```python
from build123d import *

# Parameters (mm, degrees)
F1_DEPTH = 20
F3_D     = 4.55
F4_R     = 5


with BuildPart() as f1:
    # F0 (on Right) → F1 (new body)
    with BuildSketch(Plane.YZ):
        Polygon((-15.453118, 0), (0, 0), (0, 13.234019), (-7.305924, 13.234019), (-7.305924, 2.900996), (-15.453118, 2.900996), align=None)
        Polygon((0, 13.234019), (0, 0), (15.453118, 0), (15.453118, 2.900996), (7.305924, 2.900996), (7.305924, 13.234019), align=None)
    extrude(amount=F1_DEPTH)

    # F3 (through all)
    with Locations(Plane.YZ.offset(20)):
        with Locations((0, 7.294424)):
            Hole(F3_D / 2)

    # F4
    f4_edges = [f1.edges().sort_by_distance(p)[0] for p in [
        (10, 7.305924, 13.234019),
        (10, -7.305924, 13.234019),
    ]]
    fillet(f4_edges, radius=F4_R)


solid = f1.part
```
Design review of the part built by this model. Coordinates are the model's own, in mm. A direction names the side the tool comes from. Coordinates: 2 decimals unless noted, no trailing zeros. Order: outer loops, then holes, each group sorted by start corner. A loop starts at its lowest first (then second) coordinate and runs counter-clockwise, first axis right, second up. Notation, with made-up numbers: M 65,87 L 93,87 A20 cw 93,91 Z; hole C 23.5,24 d10. An arc over 180 degrees is marked long. Answer as a JSON object with one key per item and string values. Group by question number.
1) Tool access review of faces 5 (the flat face through (10, -7.306, 6)), 6 (the flat face through (10, 11, 2.901)), 7 (the flat face through (10, -15.453, 1)): name each direction out of +Z, -Z, +X, -X, +Y, -Y from which nothing blocks a thin tool from reaching the whole face with its end or side.
2) Wall thickness on L1, parallel to Z at x = 12.25, y = 0; L2, parallel to Z at x = 18.5, y = 11.5; L3, parallel to Y at x = 12.75, z = 3.25: over which ranges is each line inside the solid? List them lowest first.
3) Add section C-C, the plane z = 6. Write out the cut boundary in (x, y).
4) Mouldability with a two-part tool opening along Z and no side actions: class faces 1 (the flat face through (10, -11, 2.901)), 2 (the flat face through (10, 0, 0)), 3 (the flat face through (20, 0, 4)), 4 (the cylindrical face through (9.86, 0.493, 5.074)) as pulls with the +Z half, pulls with the -Z half, needs draft (parallel to the pull), parting line crosses it, or undercut.
5) Add section D-D, the plane y = 12.5. Write out the cut boundary in (x, z), then the cut area to 3 significant figures.
6) Add section B-B, the plane x = 17. Write out the cut boundary in (y, z) (3 decimals), then the cut area to 3 significant figures.
7) Add section A-A, the plane y = 0. Write out the cut boundary in (x, z), then the cut area to 3 significant figures.
8) For pin 1 (4.5 mm diameter, centred on x = 9.5, z = 6, fed in from -Y); pin 2 (1.5 mm diameter, centred on y = 10, z = 7, fed in from -X); pin 3 (6 mm diameter, centred on x = 9.5, y = -11, fed in from +Z); pin 4 (5 mm diameter, centred on x = 17, y = 7.5, fed in from -Z), all flat-tipped, find the tip position at first contact; note any pin that passes through.
Computed values:
{
 "1": {"face 5": "+Z, +X, -X, -Y", "face 6": "+Z, +X, -X, +Y", "face 7": "+Z, -Z, +X, -X, -Y"},
 "2": {"L1": "z = 0 to 5.02, 9.57 to 13.23", "L2": "z = 0 to 2.9", "L3": "y = -7.31 to 7.31"},
 "3": {"outline": "M 0,-7.31 L 20,-7.31 L 20,-1.87 L 0,-1.87 Z; M 0,1.87 L 20,1.87 L 20,7.31 L 0,7.31 Z"},
 "4": {"face 1": "pulls with the +Z half", "face 2": "pulls with the -Z half", "face 3": "needs draft", "face 4": "undercut"},
 "5": {"outline": "M 0,0 L 20,0 L 20,2.9 L 0,2.9 Z", "area": "58.0 mm^2"},
 "6": {"outline": "M -15.453,0 L 15.453,0 L 15.453,2.901 L 7.306,2.901 L 7.306,8.234 A5 ccw 2.306,13.234 L -2.306,13.234 A5 ccw -7.306,8.234 L -7.306,2.901 L -15.453,2.901 Z; hole C 0,7.294 d4.55", "area": "214 mm^2"},
 "7": {"outline": "M 0,0 L 20,0 L 20,5.02 L 0,5.02 Z; M 0,9.57 L 20,9.57 L 20,13.23 L 0,13.23 Z", "area": "174 mm^2"},
 "8": {"pin 1": "stops at y = -7.31", "pin 2": "passes through", "pin 3": "stops at z = 2.9", "pin 4": "stops at z = 0"}
}
